from build123d import *

# Parameters (mm, degrees)
F1_DEPTH  = 184.15
F2_T      = -2.54
F4_DEPTH  = 2.54
F5_W      = 363.22
F5_H      = 299.72
F5_W_2    = 337.82
F5_H_2    = 274.32
F6_DEPTH  = 2.54
F7_R      = 2.5796875
F8_DEPTH  = 391.161
F9_R      = 3.175
F10_DEPTH = 2.541


with BuildPart() as f1:
    # F0 (on Right) → F1 (new body, symmetric)
    with BuildSketch(Plane.YZ):
        Polygon((47.8071639518, 50.8), (98.6071639518, 50.8), (98.6071639518, 355.6), (47.8071639518, 355.6), (-256.9928360482, 76.2), (-256.9928360482, 0), (47.8071639518, 0), align=None)
    extrude(amount=F1_DEPTH, both=True)

    # F2
    f2_openings = [f1.faces().sort_by_distance(p)[0] for p in [
        (0, 98.607164, 203.2),
        (0, -104.592836, 0),
    ]]
    offset(amount=F2_T, openings=f2_openings, kind=Kind.INTERSECTION)

    # F3 (on face) → F4 (join)
    with BuildSketch(Plane(origin=(0, 98.6071639518, 0), x_dir=(-1, 0, 0), z_dir=(0, 1, 0))):
        Polygon((-207.01, 50.8), (-181.61, 50.8), (-181.61, 353.06), (181.61, 353.06), (181.61, 50.8), (207.01, 50.8), (207.01, 378.46), (-207.01, 378.46), align=None)
    extrude(amount=-F4_DEPTH)

    # F5 (on face) → F6 (join)
    with BuildSketch(Plane.XY.offset(53.34)):
        with Locations((0, -104.5928360482)):
            Rectangle(F5_W, F5_H)
        with Locations((0, -104.5928360482)):
            Rectangle(F5_W_2, F5_H_2, mode=Mode.SUBTRACT)
    extrude(amount=-F6_DEPTH)

    # F7 (on face) → F8 (cut, through all)
    with BuildSketch(Plane(origin=(-184.15, 0, 0), x_dir=(0, -1, 0), z_dir=(-1, 0, 0))):
        with Locations((-22.4071639518, 38.1)):
            Circle(F7_R)
        with Locations((231.5928360482, 38.1)):
            Circle(F7_R)
    extrude(amount=-F8_DEPTH, mode=Mode.SUBTRACT)

    # F9 (on face) → F10 (cut, through all)
    with BuildSketch(Plane.XZ.offset(-96.0671639518)):
        with Locations((-194.31, 365.76)):
            Circle(F9_R)
        with Locations((-194.31, 314.96)):
            Circle(F9_R)
        with Locations((-194.31, 264.16)):
            Circle(F9_R)
        with Locations((-194.31, 213.36)):
            Circle(F9_R)
        with Locations((-194.31, 162.56)):
            Circle(F9_R)
        with Locations((-194.31, 111.76)):
            Circle(F9_R)
        with Locations((-194.31, 60.96)):
            Circle(F9_R)
        with Locations((196.215, 365.76)):
            Circle(F9_R)
        with Locations((196.215, 314.96)):
            Circle(F9_R)
        with Locations((196.215, 264.16)):
            Circle(F9_R)
        with Locations((196.215, 213.36)):
            Circle(F9_R)
        with Locations((196.215, 162.56)):
            Circle(F9_R)
        with Locations((196.215, 111.76)):
            Circle(F9_R)
        with Locations((196.215, 60.96)):
            Circle(F9_R)
        with Locations((147.3962, 365.76)):
            Circle(F9_R)
        with Locations((98.5774, 365.76)):
            Circle(F9_R)
        with Locations((49.7586, 365.76)):
            Circle(F9_R)
        with Locations((0.9398, 365.76)):
            Circle(F9_R)
        with Locations((-47.879, 365.76)):
            Circle(F9_R)
        with Locations((-96.6978, 365.76)):
            Circle(F9_R)
        with Locations((-145.5166, 365.76)):
            Circle(F9_R)
    extrude(amount=-F10_DEPTH, mode=Mode.SUBTRACT)


solid = f1.part
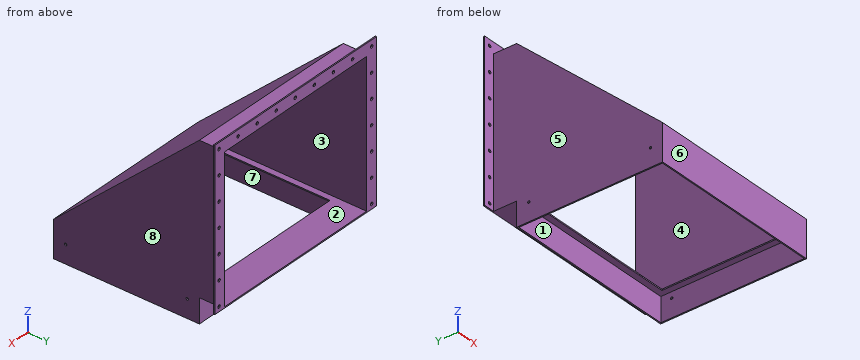
Design review of the part built by this model. Coordinates are the model's own, in mm. Face numbers are marked on the shaded views. A direction names the side the tool comes from. Round coordinates to 2 decimals unless told otherwise and drop trailing zeros. Write each loop counter-clockwise with the first axis right and the second up, starting at its lowest first coordinate (ties: lowest second). Pieces come first, ordered by that corner, then holes.
Item 1: Draft analysis for pull direction Z (two halves, no side actions). For the marked faces 1, 2 and 3, state which applies: released by +Z, released by -Z, zero draft, split by the parting line, or undercut.
Item 2: For the marked faces 4, 5, 6, 7 and 8, list the 3-axis set-ups (+Z, -Z, +X, -X, +Y, -Y) from which the entire face can be reached by the end or side of a thin tool; tool diameter is ignored.
Item 3: For pin 1 Ø11 at (x, z) = (9.5, 60.5) entering from +Y; pin 2 Ø8.5 at (x, z) = (196.215, 264.16) entering from -Y; pin 3 Ø6 at (y, z) = (22.41, 38.1) entering from -X; pin 4 Ø5.5 at (x, z) = (-47.879, 365.76) entering from +Y, all flat-tipped, find the tip position at first contact; note any pin that passes through.
Item 4: Consider section B-B on y = 74. Give the boundary of the cut face in (x, z).
Item 5: Consider section C-C on z = 83. Give the boundary of the cut face in (x, y).
Item 6: Consider section D-D on y = -33. Give the boundary of the cut face in (x, z), and give its area (3 significant figures).
Item 7: Consider section A-A on x = -135. Give the boundary of the cut face in (y, z).
Item 8: Wall thickness on L1, parallel to Y at x = -182, z = 38; L2, parallel to X at y = 97, z = 162; L3, parallel to X at y = 96.9, z = 314.96 (3 decimals): over which ranges is each line inside the solid? List them lowest first.
Check values:
1. face 1: zero draft
1. face 2: undercut
1. face 3: undercut
2. face 4: +Y
2. face 5: +Z, -Z, -X, -Y
2. face 6: +Z, -Z, +X, -X, -Y
2. face 7: -Z
2. face 8: +Z, -Z, +X, -Y
3. pin 1: stops at y = -254.45
3. pin 2: stops at y = 96.07
3. pin 3: stops at x = -184.15
3. pin 4: passes through
4. outline: (-184.15, 50.8) - (184.15, 50.8) - (184.15, 355.6) - (-184.15, 355.6) - close; hole (-181.61, 53.34) - (181.61, 53.34) - (181.61, 353.06) - (-181.61, 353.06) - close
5. outline: (-207.01, 96.07) - (-184.15, 96.07) - (-184.15, -249.57) - (184.15, -249.57) - (184.15, 96.07) - (207.01, 96.07) - (207.01, 98.61) - (181.61, 98.61) - (181.61, -245.82) - (-181.61, -245.82) - (-181.61, 98.61) - (-207.01, 98.61) - close
6. outline: (-184.15, 0) - (-181.61, 0) - (-181.61, 50.8) - (-168.91, 50.8) - (-168.91, 53.34) - (-181.61, 53.34) - (-181.61, 278.08) - (181.61, 278.08) - (181.61, 53.34) - (168.91, 53.34) - (168.91, 50.8) - (181.61, 50.8) - (181.61, 0) - (184.15, 0) - (184.15, 281.53) - (-184.15, 281.53) - close
6. area: 2,750 mm2
7. outline: (-256.99, 0) - (-254.45, 0) - (-254.45, 50.8) - (-241.75, 50.8) - (-241.75, 53.34) - (-254.45, 53.34) - (-254.45, 75.08) - (48.8, 353.06) - (98.61, 353.06) - (98.61, 378.46) - (96.07, 378.46) - (96.07, 355.6) - (47.81, 355.6) - (-256.99, 76.2) - close; (32.57, 50.8) - (45.27, 50.8) - (45.27, 0) - (47.81, 0) - (47.81, 50.8) - (98.61, 50.8) - (98.61, 53.34) - (32.57, 53.34) - close
8. L1: y = -256.99 to -234.17, -229.02 to 19.83, 24.98 to 47.81
8. L2: x = -207.01 to -197.44, -191.18 to -181.61, 181.61 to 193.09, 199.34 to 207.01
8. L3: x = -207.01 to -197.485, -191.135 to -181.61, 181.61 to 193.04, 199.39 to 207.01
